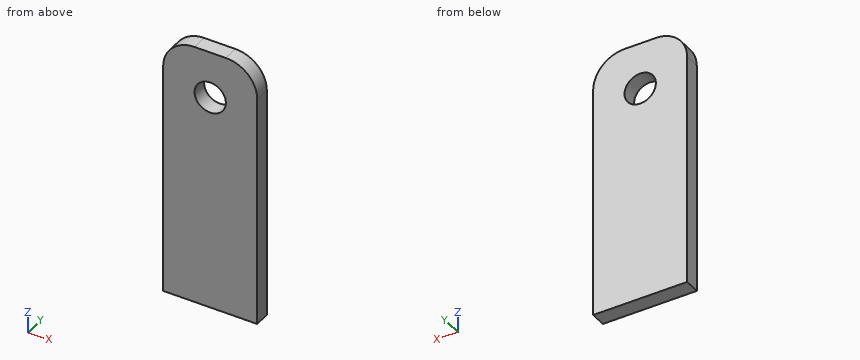
```python
from build123d import *

# Parameters (mm, degrees)
F0_W     = 30
F0_H     = 84.82
F0_R     = 5
F1_DEPTH = 5
F2_R     = 10


with BuildPart() as f1:
    # F0 (on Front) → F1 (new body)
    with BuildSketch(Plane.XZ):
        Rectangle(F0_W, F0_H)
        with Locations((0, 27.41)):
            Circle(F0_R, mode=Mode.SUBTRACT)
    extrude(amount=F1_DEPTH)

    # F2
    f2_edges = [f1.edges().sort_by_distance(p)[0] for p in [
        (15, -2.5, 42.41),
        (-15, -2.5, 42.41),
    ]]
    fillet(f2_edges, radius=F2_R)


solid = f1.part
```
Geometry check sheet. Reference: the model listing, model coordinates, mm. Give positions to 0.01 mm unless a question says otherwise; leave off trailing zeros. Order: outer loops, then holes, each group sorted by start corner. A loop starts at its lowest first (then second) coordinate and runs counter-clockwise, first axis right, second up. Notation, with made-up numbers: (-11, 85) - (0, 85) arc R26 ccw to (0, 110) - close; hole circle Ø2 at (85, 20). An arc over 180 degrees is marked (long way). Write item = value, one per line. Start each with the question number.
1) Scan lines: L1, parallel to Z at x = 0, y = -1.7; L2, parallel to Z at x = -4.5, y = -4.35; L3, parallel to Z at x = -10, y = -2.9. Record each from-to range of solid material in increasing order.
2) Section check B-B (y = -4). Enter the section's corners in (x, z).
3) Section check C-C (z = 27.41). Enter the section's corners in (x, y), then the cut area to 3 significant figures.
4) Section check D-D (x = -13). Enter the section's corners in (y, z), then the cut area to 3 significant figures.
5) Section check A-A (x = 4). Enter the section's corners in (y, z).
6) Gauge pin test, flat ends, axial feed: pin 1 Ø2 at (x, y) = (8.5, -3.5) entering from +Z; pin 2 Ø1 at (x, y) = (10.5, -1) entering from +Z. Record the tip position at first contact, or that the pin passes through.
Geometry check:
q1.L1 = -42.41 to 22.41, 32.41 to 42.41
q1.L2 = -42.41 to 25.23, 29.59 to 42.41
q1.L3 = -42.41 to 41.07
q2.outline = (-15, -42.41) - (15, -42.41) - (15, 32.41) arc R10 ccw to (5, 42.41) - (-5, 42.41) arc R10 ccw to (-15, 32.41) - close; hole circle Ø10 at (0, 27.41)
q3.outline = (-15, -5) - (-5, -5) - (-5, 0) - (-15, 0) - close; (5, -5) - (15, -5) - (15, 0) - (5, 0) - close
q3.area = 100 mm2
q4.outline = (-5, -42.41) - (0, -42.41) - (0, 38.41) - (-5, 38.41) - close
q4.area = 404 mm2
q5.outline = (-5, -42.41) - (0, -42.41) - (0, 24.41) - (-5, 24.41) - close; (-5, 30.41) - (0, 30.41) - (0, 42.41) - (-5, 42.41) - close
q6.pin_1 = 42.09
q6.pin_2 = 41.07
